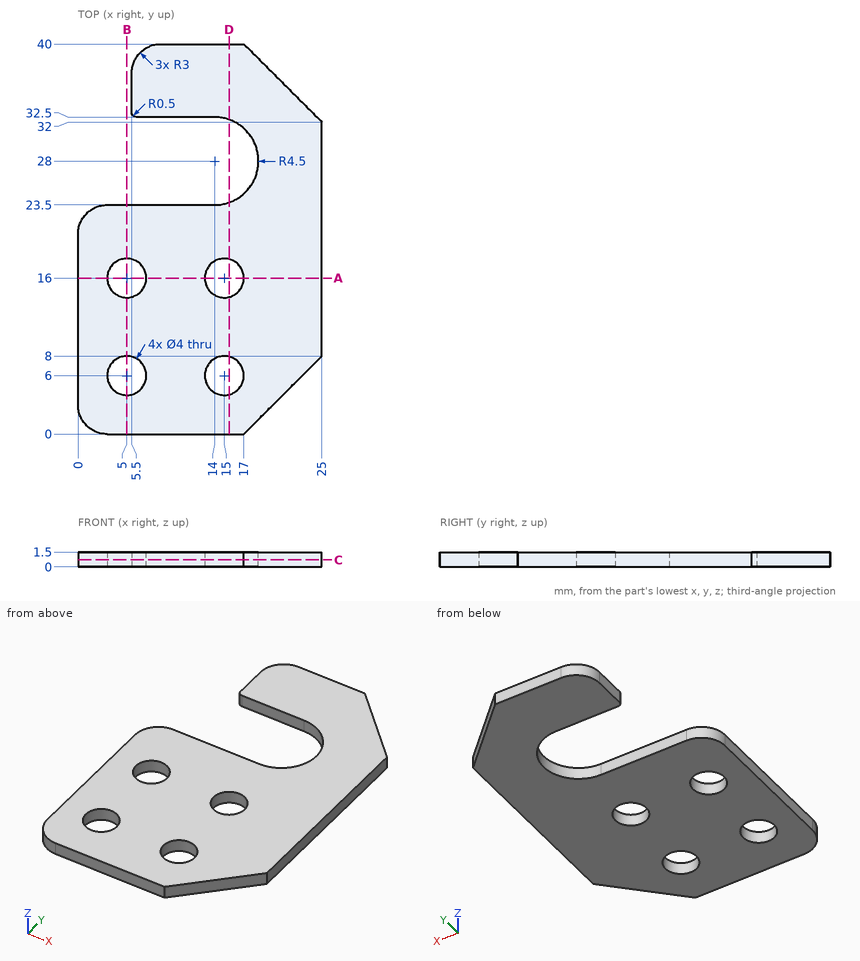
For this review, use the dimensioned drawing (mm, ordinates from the lowest corner) and the shaded views. Give positions to 0.01 mm unless a question says otherwise; leave off trailing zeros. Order: outer loops, then holes, each group sorted by start corner. A loop starts at its lowest first (then second) coordinate and runs counter-clockwise, first axis right, second up. Notation, with made-up numbers: M 38.25,39.5 L 78.25,39.5 A23 ccw 78.25,72.5 Z; hole C 73.25,50.25 d10. An arc over 180 degrees is marked long. Use one line per item in the form item = value. Start each with the question number.
Item 1: To check wall thickness, follow line 1 along Y through (x, z) = (5, 0.7); line 2 along Y through (x, z) = (11.5, 0.1); line 3 along Y through (x, z) = (16.5, 0.3). State the ranges of each line that lie inside material, in increasing order. Write a range as from..to.
Item 2: We need section B-B on x = 5. Give the boundary of the cut face in (y, z), plus the area to 4 significant figures.
Item 3: We need section D-D on x = 15.5. Give the boundary of the cut face in (y, z).
Item 4: Insertion check: pin 1 Ø6.5 at (x, y) = (5, 16) entering from +Z. The pin has a flat end and moves straight along its axis. Give the tip position at first contact, or say it passes through.
Item 5: We need section C-C on z = 0.7. Give the boundary of the cut face in (x, y).
Item 6: We need section A-A on y = 16. Give the boundary of the cut face in (x, z), plus the area to 3 significant figures.
Completed:
q1.line_1 = 0..4, 8..14, 18..23.5
q1.line_2 = 0..23.5, 32.5..40
q1.line_3 = 0..4.68, 7.32..14.68, 17.32..24.26, 31.74..40
q2.outline = M 0,0 L 4,0 L 4,1.5 L 0,1.5 Z; M 8,0 L 14,0 L 14,1.5 L 8,1.5 Z; M 18,0 L 23.5,0 L 23.5,1.5 L 18,1.5 Z
q2.area = 23.25 mm²
q3.outline = M 0,0 L 4.06,0 L 4.06,1.5 L 0,1.5 Z; M 7.94,0 L 14.06,0 L 14.06,1.5 L 7.94,1.5 Z; M 17.94,0 L 23.76,0 L 23.76,1.5 L 17.94,1.5 Z; M 32.24,0 L 40,0 L 40,1.5 L 32.24,1.5 Z
q4.pin_1 = 1.5
q5.outline = M 0,3 A3 ccw 3,0 L 17,0 L 25,8 L 25,32 L 17,40 L 8.5,40 A3 ccw 5.5,37 L 5.5,33 A0.5 ccw 6,32.5 L 14,32.5 A4.5 cw 14,23.5 L 3,23.5 A3 ccw 0,20.5 Z; hole C 5,6 d4; hole C 5,16 d4; hole C 15,6 d4; hole C 15,16 d4
q6.outline = M 0,0 L 3,0 L 3,1.5 L 0,1.5 Z; M 7,0 L 13,0 L 13,1.5 L 7,1.5 Z; M 17,0 L 25,0 L 25,1.5 L 17,1.5 Z
q6.area = 25.5 mm²
